The listing builds one solid part. Answer for the finished solid, in the listing's coordinates (mm). A direction names the side the tool comes from. Give positions to 0.01 mm unless a question says otherwise; leave off trailing zeros. Write each loop counter-clockwise with the first axis right and the second up, starting at its lowest first coordinate (ties: lowest second). Pieces come first, ordered by that corner, then holes. Notation, with made-up numbers: M 5.5,-4.75 L 28.5,-4.75 A24 ccw 28.5,11.25 Z; hole C 60,34 d7. An arc over 180 degrees is marked long. Answer as a JSON object with one key per item and string values.
```python
from build123d import *

# Parameters (mm, degrees)
F0_R     = 15
F1_DEPTH = 5
F3_DEPTH = 25


with BuildPart() as f1:
    # F0 (on Top) → F1 (new body)
    with BuildSketch(Plane.XY):
        Circle(F0_R)
        Polygon((-2.8688276582, 13.7029131161), (10.4326570353, 9.3359341892), (13.3014846935, -4.3669789269), (2.8688276582, -13.7029131161), (-10.4326570353, -9.3359341892), (-13.3014846935, 4.3669789269), align=None, mode=Mode.SUBTRACT)
        Polygon((13.3014846935, -4.3669789269), (10.4326570353, 9.3359341892), (-2.8688276582, 13.7029131161), (-13.3014846935, 4.3669789269), (-10.4326570353, -9.3359341892), (2.8688276582, -13.7029131161), align=None)
    extrude(amount=F1_DEPTH)

    # F2 (on face) → F3 (cut)
    with BuildSketch(Plane(origin=(0, 0, 0), x_dir=(1, 0, 0), z_dir=(0, 0, -1))):
        Polygon((-13.1988527334, 4.668006697), (-10.6420387513, -9.0965384194), (2.5568139821, -13.7645451164), (13.1988527334, -4.668006697), (10.6420387513, 9.0965384194), (-2.5568139821, 13.7645451164), align=None)
    extrude(amount=-F3_DEPTH, mode=Mode.SUBTRACT)


solid = f1.part
```
1. Consider line 1 along X through (y, z) = (2.25, 4.05); line 2 along X through (y, z) = (0.25, 2.75); line 3 along Y through (x, z) = (-8.5, 4.35). Determine where each line is inside the solid, lowest interval first.
Verdict:
{"line 1": "x = -14.83 to -11.91, 12.75 to 14.83", "line 2": "x = -15 to -12.29, 12.38 to 15", "line 3": "y = -12.36 to -8.68, 9.85 to 12.36"}
2. Flat-ended cylindrical pins translate along their axes: pin 1 (5 mm diameter, centred on x = 8, y = 5.5, fed in from +Z); pin 2 (2 mm diameter, centred on y = 6.5, z = 3, fed in from -X); pin 3 (1 mm diameter, centred on y = 7, z = 3.5, fed in from +X); pin 4 (2 mm diameter, centred on y = -2, z = 4, fed in from +X). Find the tip coordinate at first contact, or state that the pin passes through.
Verdict:
{"pin 1": "passes through", "pin 2": "stops at x = -13.96", "pin 3": "stops at x = 13.52", "pin 4": "stops at x = 14.97"}
3. A cutting plane is placed at B-B, the plane y = 0. Give the vertices of the cut face in (x, z), plus the area to 3 significant figures.
Verdict:
{"outline": "M -15,0 L -12.33,0 L -12.33,5 L -15,5 Z; M 12.33,0 L 15,0 L 15,5 L 12.33,5 Z", "area": "26.7 mm2"}
4. A cutting plane is placed at C-C, the plane z = 1.5. Give the vertices of the cut face in (x, y).
Verdict:
{"outline": "C 0,0 d30; hole M -13.2,-4.67 L -2.56,-13.76 L 10.64,-9.1 L 13.2,4.67 L 2.56,13.76 L -10.64,9.1 Z"}
5. The mould has two halves that part along Y. Classify faces 1 (the flat face through (-7.803, -9.28, 2.465)), 2 (the cylindrical face through (-14.985, 0.66, 2.465)), 3 (the flat face through (-8, -10, 5)): released by +Y, released by -Y, zero draft, split by the parting line, or undercut.
Verdict:
{"face 1": "undercut", "face 2": "split by the parting line", "face 3": "zero draft"}
6. For faces 4 (the flat face through (-8, -10, 0)), 5 (the flat face through (-11.938, 2.118, 2.465)), determine the directions among +Z, -Z, +X, -X, +Y, -Y from which every point of the face is accessible in a straight line to the end or side of a thin tool.
Verdict:
{"face 4": "-Z, +X, -X, +Y, -Y", "face 5": "+Z, -Z"}
7. A cutting plane is placed at A-A, the plane x = 11.5. Give the vertices of the cut face in (y, z), plus the area to 3 significant figures.
Verdict:
{"outline": "M -9.63,0 L -4.48,0 L -4.48,5 L -9.63,5 Z; M 6.12,0 L 9.63,0 L 9.63,5 L 6.12,5 Z", "area": "43.3 mm2"}
